Read the model definition and answer for the solid it produces. Units are mm, in the model's axes. Face numbers are marked on the shaded views. A direction names the side the tool comes from. Round coordinates to 2 decimals unless told otherwise and drop trailing zeros. Loops run counter-clockwise (first coordinate to the right, second up) from the corner with the lowest first, then second, coordinate; pieces in that order, holes last. Notation, with made-up numbers: (31, 62.5) - (80, 62.5) arc R27 cw to (80, 96.5) - close; hole circle Ø9 at (30.25, -34.5). An arc over 180 degrees is marked (long way). Use CSV: the item, a comma, the result in double quotes. Start each with the question number.
1. Find section D-D (z = 66). Give the vertices of the cut face in (x, y).
2. Find section C-C (x = -9). Give the vertices of the cut face in (y, z).
3. Find section A-A (y = 0). Give the vertices of the cut face in (x, z).
4. Consider line 1 along Y through (x, z) = (69, -7); line 2 along Z through (x, y) = (14.5, 32.5); line 3 along X through (y, z) = (2, 7). Determine where each line is inside the solid, lowest interval first.
5. Find section B-B (y = 43). Give the vertices of the cut face in (x, z), and give its area (3 significant figures).
6. A tool of negligible diameter and unlimited length cuts with its end or side. For the marked faces 1 and 2, from which of +Z, -Z, +X, -X, +Y, -Y can it reach the whole face along a straight path? Write none if from no direction.
from build123d import *

# Parameters (mm, degrees)
F0_W     = 228.6
F0_H     = 152.4
F1_DEPTH = 76.2
F2_W     = 152.433592
F2_H     = 76.2
F3_DEPTH = 152.401
F5_D     = 25.4


with BuildPart() as f1:
    # F0 (on Front) → F1 (new body, symmetric)
    with BuildSketch(Plane.XZ):
        with Locations((6.091539, 0)):
            Rectangle(F0_W, F0_H)
    extrude(amount=F1_DEPTH, both=True)

    # F2 (on face) → F3 (cut, through all)
    with BuildSketch(Plane.XZ.offset(76.2)):
        with Locations((44.174743, 38.1)):
            Rectangle(F2_W, F2_H)
    extrude(amount=-F3_DEPTH, mode=Mode.SUBTRACT)

    # F5 (through all)
    with Locations(Plane.XY):
        with Locations((69.591539, 0)):
            Hole(F5_D / 2)


solid = f1.part
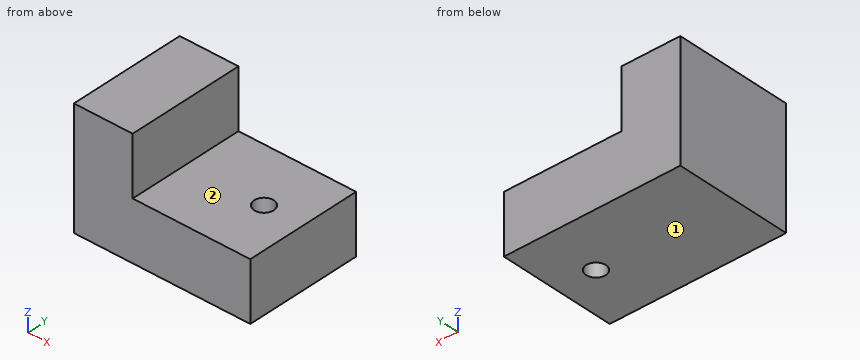
Filled sheet:
1,outline,"(-108.21, -76.2) - (-32.04, -76.2) - (-32.04, 76.2) - (-108.21, 76.2) - close"
2,outline,"(-76.2, -76.2) - (76.2, -76.2) - (76.2, 0) - (-76.2, 0) - close"
3,outline,"(-108.21, -76.2) - (56.89, -76.2) - (56.89, 0) - (-32.04, 0) - (-32.04, 76.2) - (-108.21, 76.2) - close; (82.29, -76.2) - (120.39, -76.2) - (120.39, 0) - (82.29, 0) - close"
4,line 1,"y = -76.2 to -12.69, 12.69 to 76.2"
4,line 2,"z = -76.2 to 0"
4,line 3,"x = -108.21 to -32.04"
5,outline,"(-108.21, -76.2) - (120.39, -76.2) - (120.39, 0) - (-32.04, 0) - (-32.04, 76.2) - (-108.21, 76.2) - close"
5,area,"23,200 mm²"
6,face 1,"-Z, +X, -X, +Y, -Y"
6,face 2,"+Z, +X, +Y, -Y"
